```python
from build123d import *

# Parameters (mm, degrees)
EXTRUDE_1_DEPTH          = 85
SKETCH_2_R               = 58
EXTRUDE_2_DEPTH          = 5
SKETCH_3_R               = 40
CUT_EXTRUDE_1_DEPTH      = 44
SKETCH_4_R               = 35
CUT_EXTRUDE_2_DEPTH      = 187.38937738
PATTERN_CIRCULAR_1_COUNT = 6
SKETCH_8_W               = 120
SKETCH_8_H               = 36
CUT_EXTRUDE_3_DEPTH      = 200.624647777


with BuildPart() as part:
    # 草图1 → 凸台-拉伸1 (new body)
    with BuildSketch(Plane.XY):
        Polygon((0, 0), (-57, 0), (-57, 18), (-135, 18), (-135, 58), (-60, 58), (-60, 120), (60, 120), (60, 58), (135, 58), (135, 18), (57, 18), (57, 0), align=None)
    extrude(amount=-EXTRUDE_1_DEPTH)

    # 草图2 → 凸台-拉伸2 (add)
    with BuildSketch(Plane.XY):
        with Locations((0, 60)):
            Circle(SKETCH_2_R)
    extrude(amount=EXTRUDE_2_DEPTH)

    # 草图3 → 切除-拉伸1 (cut)
    with BuildSketch(Plane.XY.offset(5)):
        with Locations((0, 60)):
            Circle(SKETCH_3_R)
    extrude(amount=-CUT_EXTRUDE_1_DEPTH, mode=Mode.SUBTRACT)

    # 草图4 → 切除-拉伸2 (cut, through all)
    with BuildSketch(Plane.XY.offset(-39)):
        with Locations((0, 60)):
            Circle(SKETCH_4_R)
    extrude(amount=-CUT_EXTRUDE_2_DEPTH, mode=Mode.SUBTRACT)

    # 草图7 → M8 螺纹孔1 (revolve, cut)
    with BuildSketch(Plane(origin=(24, 101.569219382, 5), x_dir=(0, -1, 0), z_dir=(1, 0, 0))):
        Polygon((0, 0), (0, 29.802926105), (3.4, 27.76), (3.4, 0), align=None)
    hole_wizard_m8_1 = revolve(axis=Axis((24, 101.569219382, 11.35), (0, 0, -1)), mode=Mode.SUBTRACT)

    # 阵列(圆周)1: M8 螺纹孔1 ×6 about axis
    pattern_circular_1_axis = Axis((0, 60, 0), (0, 0, 1))
    for i in range(1, PATTERN_CIRCULAR_1_COUNT):
        add(hole_wizard_m8_1.rotate(pattern_circular_1_axis, i * 360 / PATTERN_CIRCULAR_1_COUNT), mode=Mode.SUBTRACT)

    # 草图8 → 切除-拉伸3 (cut, through all)
    with BuildSketch(Plane(origin=(0, 120, 0), x_dir=(1, 0, 0), z_dir=(0, 1, 0))):
        with Locations((0, 67)):
            Rectangle(SKETCH_8_W, SKETCH_8_H)
    extrude(amount=-CUT_EXTRUDE_3_DEPTH, mode=Mode.SUBTRACT)


solid = part.part
```
Geometry check sheet. Reference: the model listing, model coordinates, mm. A direction names the side the tool comes from. Give positions to 0.01 mm unless a question says otherwise; leave off trailing zeros. Write each loop counter-clockwise with the first axis right and the second up, starting at its lowest first coordinate (ties: lowest second). Pieces come first, ordered by that corner, then holes. Notation, with made-up numbers: (48.25, 22) -> (77.25, 22) arc R14 ccw to (77.25, 36) -> close; hole circle Ø8 at (18.5, 27.25). An arc over 180 degrees is marked (long way). One line per question, with ' | ' between items.
Item 1: Sectioned sample at A-A, the plane z = -79. Record the boundary of the cut face in (x, y), plus the area to 3 significant figures.
Determined:
outline: (-135, 18) -> (-60, 18) -> (-60, 58) -> (-135, 58) -> close; (60, 18) -> (135, 18) -> (135, 58) -> (60, 58) -> close | area: 6,000 mm^2
Item 2: Sectioned sample at D-D, the plane z = -13. Record the boundary of the cut face in (x, y).
Determined:
outline: (-135, 18) -> (-57, 18) -> (-57, 0) -> (57, 0) -> (57, 18) -> (135, 18) -> (135, 58) -> (60, 58) -> (60, 120) -> (-60, 120) -> (-60, 58) -> (-135, 58) -> close; hole circle Ø6.8 at (-48, 60); hole circle Ø80 at (0, 60); hole circle Ø6.8 at (-24, 18.43); hole circle Ø6.8 at (-24, 101.57); hole circle Ø6.8 at (24, 18.43); hole circle Ø6.8 at (24, 101.57); hole circle Ø6.8 at (48, 60)
Item 3: Sectioned sample at B-B, the plane x = -1.5. Record the boundary of the cut face in (y, z).
Determined:
outline: (0, -49) -> (25.03, -49) -> (25.03, -39) -> (20.03, -39) -> (20.03, 5) -> (2.02, 5) -> (2.02, 0) -> (0, 0) -> close; (94.97, -49) -> (120, -49) -> (120, 0) -> (117.98, 0) -> (117.98, 5) -> (99.97, 5) -> (99.97, -39) -> (94.97, -39) -> close
Item 4: Access from +Z, -Z, +X, -X, +Y, -Y to the whole of each face (thin tool, end or side, straight path). Record for faces 1 (the flat face through (60, 38, -67)), 2 (the flat face through (97, 58, -42)), 3 (the flat face through (-0.2, 24.6, -39)), 4 (the flat face through (-57, 9, -24)).
Determined:
face 1: -Z, +Y, -Y | face 2: +Z, -Z, +X, +Y | face 3: +Z | face 4: +Z, -Z, -X, -Y
Item 5: Sectioned sample at C-C, the plane y = 68.5. Record the boundary of the cut face in (x, z), plus the area to 3 significant figures.
Determined:
outline: (-60, -49) -> (-33.95, -49) -> (-33.95, -39) -> (-39.09, -39) -> (-39.09, 5) -> (-57.37, 5) -> (-57.37, 0) -> (-60, 0) -> close; (33.95, -49) -> (60, -49) -> (60, 0) -> (57.37, 0) -> (57.37, 5) -> (39.09, 5) -> (39.09, -39) -> (33.95, -39) -> close | area: 2,340 mm^2
Item 6: Depth check by flat-ended pin: pin 1 (1.5 mm diameter, centred on x = -88, z = -39, fed in from +Y); pin 2 (5 mm diameter, centred on x = -64.5, z = -67.5, fed in from -Y); pin 3 (24.5 mm diameter, centred on y = 101, z = -25, fed in from -X); pin 4 (6 mm diameter, centred on x = 55, z = -71, fed in from -Y). Enter the tip coordinate at first touch or a pass-through.
Determined:
pin 1: y = 58 | pin 2: y = 18 | pin 3: x = -60 | pin 4: through
Item 7: Scan lines: line 1 along Y through (x, z) = (122.5, -59); line 2 along Y through (x, z) = (-48, -16.25); line 3 along X through (y, z) = (17, -28.5). Record each from-to range of solid material in increasing order.
Determined:
line 1: 18 to 58 | line 2: 0 to 56.6, 63.4 to 120 | line 3: -57 to 57
Item 8: Draft check along Y on faces 5 (the flat face through (10.6, 2.5, 0)), 6 (the flat face through (-1, 0, -24)), 7 (the cylindrical face through (-4.56, 94.7, -43.93)). Enter one of: released by +Y, released by -Y, zero draft, split by the parting line, or undercut.
Determined:
face 5: zero draft | face 6: released by -Y | face 7: undercut
